Source: CAD feature listing. Evaluate the final solid. Frame: model axes, mm. A direction names the side the tool comes from. Coordinates: 2 decimals unless noted, no trailing zeros. Write each loop counter-clockwise with the first axis right and the second up, starting at its lowest first coordinate (ties: lowest second). Pieces come first, ordered by that corner, then holes. Notation, with made-up numbers: (31.25, 8.5) - (43.25, 8.5) arc R18 cw to (43.25, 34.5) - close; hole circle Ø10 at (40, -40). An arc over 180 degrees is marked (long way). One line per question, with ' | ' between items.
from build123d import *

# Parameters (mm, degrees)
SKETCH1_R                = 50
BOSS_EXTRUDE1_DEPTH      = 50
BOSS_EXTRUDE2_REACH      = 227.444
BOSS_EXTRUDE2_END_RADIUS = 65
SKETCH2_R                = 45
SKETCH2_R_2              = 5
SCALE_1_SCALE            = 0.135064935


with BuildPart() as part:
    # Sketch1 → Boss-Extrude1 (new, symmetric)
    with BuildSketch(Plane.XY):
        with BuildLine():
            Line((-40, 90), (40, 90))
            Line((40, 90), (62.047471254, 19.367790554))
            ThreePointArc((62.047471254, 19.367790554), (0, -65), (-62.047471254, 19.367790554))
            Line((-62.047471254, 19.367790554), (-40, 90))
        make_face()
        with Locations(Location((0, 0, 0), (0, 0, 180))):
            Circle(SKETCH1_R, mode=Mode.SUBTRACT)
    extrude(amount=BOSS_EXTRUDE1_DEPTH, both=True)

    # Boss-Extrude2: up to this cylinder (the profile starts outside it)
    boss_extrude2_end = Plane(origin=(0, 0, 0), z_dir=(0, 0, -1)) * Cylinder(BOSS_EXTRUDE2_END_RADIUS, 585.888, mode=Mode.PRIVATE)
    # Sketch2 → Boss-Extrude2 (add, up to the surface)
    with BuildSketch(Plane(origin=(0, -120, 0), x_dir=(1, 0, 0), z_dir=(0, 1, 0)), mode=Mode.PRIVATE) as boss_extrude2_sk1:
        with Locations(Location((0, 0, 0), (0, 0, 90))):
            Circle(SKETCH2_R)
        with Locations(Location((0, 37, 0), (0, 0, 90))):
            Circle(SKETCH2_R_2, mode=Mode.SUBTRACT)
        with Locations(Location((32.04293994, 18.5, 0), (0, 0, 90))):
            Circle(SKETCH2_R_2, mode=Mode.SUBTRACT)
        with Locations(Location((32.04293994, -18.5, 0), (0, 0, 90))):
            Circle(SKETCH2_R_2, mode=Mode.SUBTRACT)
        with Locations(Location((0, -37, 0), (0, 0, 90))):
            Circle(SKETCH2_R_2, mode=Mode.SUBTRACT)
        with Locations(Location((-32.04293994, -18.5, 0), (0, 0, 90))):
            Circle(SKETCH2_R_2, mode=Mode.SUBTRACT)
        with Locations(Location((-32.04293994, 18.5, 0), (0, 0, 90))):
            Circle(SKETCH2_R_2, mode=Mode.SUBTRACT)
    boss_extrude2_tool1 = extrude(boss_extrude2_sk1.sketch, amount=BOSS_EXTRUDE2_REACH, mode=Mode.PRIVATE) - boss_extrude2_end
    add(boss_extrude2_tool1.solids().sort_by_distance((0, -120, 0))[0])


with BuildPart() as part_1:
    # 缩放比例1: scaled about (6.7865e-05, -8.166687409, 3.34e-07)
    add(part.part.scale(SCALE_1_SCALE).moved(Location((5.8699e-05, -7.063654304, 2.89e-07))))


solid = part_1.part
Item 1: Cut plane A-A on y = -5.75. Return loops of the section in (x, z).
Check sheet entries:
outline: (-8.68, -6.75) - (-6.62, -6.75) - (-6.62, 6.75) - (-8.68, 6.75) - close; (6.62, -6.75) - (8.68, -6.75) - (8.68, 6.75) - (6.62, 6.75) - close
Item 2: Cut plane B-B on x = 1.5. Return loops of the section in (y, z).
Check sheet entries:
outline: (-23.27, -5.89) - (-15.71, -5.89) - (-15.71, -6.75) - (-13.65, -6.75) - (-13.65, 6.75) - (-15.71, 6.75) - (-15.71, 5.89) - (-23.27, 5.89) - close; (-0.48, -6.75) - (5.09, -6.75) - (5.09, 6.75) - (-0.48, 6.75) - close
Item 3: Access query for faces 4 (the face through (0.88, -13.76, -0.09)), 5 (the face through (-4.997, -18.836, 2.587)). Directions: +Z, -Z, +X, -X, +Y, -Y. A direction counts if a zero-diameter tool reaches every point of the face in a straight line with its end or side. Return the directions, or none.
Check sheet entries:
face 4: +Z, -Z | face 5: -Y
Item 4: Ray query, line 1 along Y through (x, z) = (0.25, 3); line 2 along X through (y, z) = (-7, -1.5); line 3 along X through (y, z) = (-7.5, -0.75). Return the intervals inside material, ascending. Write a range as [from, to].
Check sheet entries:
line 1: [-23.27, -13.81], [-0.32, 5.09] | line 2: [-8.78, -6.75], [6.75, 8.78] | line 3: [-8.77, -6.74], [6.74, 8.77]
Item 5: Cut plane C-C on z = 0. Return loops of the section in (x, y).
Check sheet entries:
outline: (-8.38, -4.45) arc R8.78 ccw to (-6.08, -13.4) - (-6.08, -23.27) - (6.08, -23.27) - (6.08, -13.4) arc R8.78 ccw to (8.38, -4.45) - (5.4, 5.09) - (-5.4, 5.09) - close; hole circle Ø13.51 at (0, -7.06)
Item 6: Pin query (flat end, axial travel): pin 1 Ø1.1 at (x, z) = (4.33, -2.5) entering from -Y; pin 2 Ø4 at (y, z) = (-15, 1) entering from -X; pin 3 Ø1.5 at (x, y) = (4, -16) entering from -Z. Return the tip coordinate at first contact, or that it passes through.
Check sheet entries:
pin 1: y = -14.99 | pin 2: x = -6.47 | pin 3: z = -5.14
Item 7: Mould query, pull axis Z, two halves, no side actions, for faces 1 (the face through (-0.203, -19.596, 4.353)), 2 (the face through (3.7, -18.4, 4.82)), 3 (the face through (0, 5.092, 0)). Classes: pulls with the +Z half, pulls with the -Z half, needs draft (parallel to the pull), parting line crosses it, or undercut.
Check sheet entries:
face 1: undercut | face 2: parting line crosses it | face 3: needs draft
Item 8: Cut plane D-D on y = -16.25. Return loops of the section in (x, z), and give its area (3 significant figures).
Check sheet entries:
outline: circle Ø12.16 at (0, 0); hole circle Ø1.35 at (-4.33, -2.5); hole circle Ø1.35 at (-4.33, 2.5); hole circle Ø1.35 at (0, -5); hole circle Ø1.35 at (0, 5); hole circle Ø1.35 at (4.33, -2.5); hole circle Ø1.35 at (4.33, 2.5) | area: 107 mm²
